Design review of the part built by this model. Coordinates are the model's own, in mm. Face numbers are marked on the shaded views. Give positions to 0.01 mm unless a question says otherwise; leave off trailing zeros. Write each loop counter-clockwise with the first axis right and the second up, starting at its lowest first coordinate (ties: lowest second). Pieces come first, ordered by that corner, then holes.
```python
from build123d import *

# Parameters (mm, degrees)
BASPROSKE_W         = 10
BASPROSKE_H         = 6
TOOTHCUT_DEPTH      = 14.114877049
TEETHCUTS_COUNT     = 10
TEETHCUTS_ANGLE     = 324
BORSKE_R            = 2.5
BORE_DEPTH          = 50.0000508
SKETCH1_R           = 2.5
BOSS_EXTRUDE1_DEPTH = 10
CUT_EXTRUDE2_DEPTH  = 10
CUT_EXTRUDE4_DEPTH  = 12.8
CUT_EXTRUDE5_DEPTH  = 7


with BuildPart() as part:
    # BasProSke → Base-Revolve (revolve)
    with BuildSketch(Plane(origin=(0, 0, 0), x_dir=(1, 0, 0), z_dir=(0, 1, 0)), mode=Mode.PRIVATE) as base_revolve_sk:
        with Locations((5, 3)):
            Rectangle(BASPROSKE_W, BASPROSKE_H)
    revolve(base_revolve_sk.sketch.rotate(Axis((-10, 0, 0), (1, 0, 0)), 180), axis=Axis((-10, 0, 0), (1, 0, 0)))

    # TooCutSke → ToothCut (cut, through all)
    with BuildSketch(Plane(origin=(0, 0, 0), x_dir=(0, 0, -1), z_dir=(1, 0, 0))):
        with BuildLine():
            ThreePointArc((0.59278292, 3.701838653), (0, 3.749), (-0.59278292, 3.701838653))
            ThreePointArc((-0.59278292, 3.701838653), (-0.846593509, 4.924114224), (-1.775771316, 5.757784417))
            ThreePointArc((-1.775771316, 5.757784417), (0, 6.0254), (1.775771316, 5.757784417))
            ThreePointArc((1.775771316, 5.757784417), (0.846593509, 4.924114224), (0.59278292, 3.701838653))
        make_face()
    toothcut = extrude(amount=TOOTHCUT_DEPTH, mode=Mode.SUBTRACT)

    # TeethCuts: ToothCut ×10 about axis
    teethcuts_axis = Axis((-10, 0, 0), (1, 0, 0))
    for i in range(1, TEETHCUTS_COUNT):
        add(toothcut.rotate(teethcuts_axis, i * TEETHCUTS_ANGLE / (TEETHCUTS_COUNT - 1)), mode=Mode.SUBTRACT)

    # BorSke → Bore (cut, symmetric)
    with BuildSketch(Plane(origin=(0, 0, 0), x_dir=(0, 0, -1), z_dir=(1, 0, 0))):
        with Locations(Location((0, 0, 0), (0, 0, 180))):
            Circle(BORSKE_R)
    extrude(amount=BORE_DEPTH, both=True, mode=Mode.SUBTRACT)

    # Sketch1 → Boss-Extrude1 (add)
    with BuildSketch(Plane(origin=(10, 0, 0), x_dir=(0, 0, -1), z_dir=(1, 0, 0))):
        Circle(SKETCH1_R)
    extrude(amount=-BOSS_EXTRUDE1_DEPTH)

    # Sketch2 → Cut-Extrude2 (cut)
    with BuildSketch(Plane.ZY):
        with BuildLine():
            Line((1.187434209, 2.2), (-1.187434209, 2.2))
            ThreePointArc((-1.187434209, 2.2), (-1.280900948, -2.146926352), (2.5, 0))
            ThreePointArc((2.5, 0), (2.146926352, 1.280900948), (1.187434209, 2.2))
        make_face()
    extrude(amount=-CUT_EXTRUDE2_DEPTH, mode=Mode.SUBTRACT)

    # Sketch3 → Cut-Extrude4 (cut)
    with BuildSketch(Plane.ZY):
        with BuildLine():
            ThreePointArc((-1.385640646, 2.2), (0, -2.6), (1.385640646, 2.2))
            Line((1.385640646, 2.2), (-1.385640646, 2.2))
        make_face()
    extrude(amount=-CUT_EXTRUDE4_DEPTH, mode=Mode.SUBTRACT)

    # Sketch4 → Cut-Extrude5 (cut)
    with BuildSketch(Plane(origin=(10, 0, 0), x_dir=(0, 0, -1), z_dir=(1, 0, 0))):
        with BuildLine():
            ThreePointArc((5.99882193, 0.11889261), (4.925863873, 0.720361677), (3.703837769, 0.580160996))
            ThreePointArc((3.703837769, 0.580160996), (3.56551088, 1.158504712), (3.337477777, 1.707701113))
            ThreePointArc((3.337477777, 1.707701113), (4.408525556, 2.3125653), (4.92303221, 3.429832919))
            ThreePointArc((4.92303221, 3.429832919), (4.854101966, 3.526711514), (4.783265565, 3.622205204))
            ThreePointArc((4.783265565, 3.622205204), (3.561689615, 3.478134978), (2.655457622, 2.646421322))
            ThreePointArc((2.655457622, 2.646421322), (2.203606911, 3.033004712), (1.69631471, 3.343279438))
            ThreePointArc((1.69631471, 3.343279438), (2.207280316, 4.462170935), (1.966811514, 5.668478849))
            ThreePointArc((1.966811514, 5.668478849), (1.854101966, 5.706339098), (1.740664331, 5.741958524))
            ThreePointArc((1.740664331, 5.741958524), (0.837070982, 4.907378935), (0.59278292, 3.701838653))
            ThreePointArc((0.59278292, 3.701838653), (0, 3.749), (-0.59278292, 3.701838653))
            ThreePointArc((-0.59278292, 3.701838653), (-0.837070982, 4.907378935), (-1.740664331, 5.741958524))
            ThreePointArc((-1.740664331, 5.741958524), (-1.854101966, 5.706339098), (-1.966811514, 5.668478849))
            ThreePointArc((-1.966811514, 5.668478849), (-2.207280316, 4.462170935), (-1.69631471, 3.343279438))
            ThreePointArc((-1.69631471, 3.343279438), (-2.203606911, 3.033004712), (-2.655457622, 2.646421322))
            ThreePointArc((-2.655457622, 2.646421322), (-3.561689615, 3.478134978), (-4.783265565, 3.622205204))
            ThreePointArc((-4.783265565, 3.622205204), (-4.854101966, 3.526711514), (-4.92303221, 3.429832919))
            ThreePointArc((-4.92303221, 3.429832919), (-4.408525556, 2.3125653), (-3.337477777, 1.707701113))
            ThreePointArc((-3.337477777, 1.707701113), (-3.56551088, 1.158504712), (-3.703837769, 0.580160996))
            ThreePointArc((-3.703837769, 0.580160996), (-4.925863873, 0.720361677), (-5.99882193, 0.11889261))
            ThreePointArc((-5.99882193, 0.11889261), (-6, 0), (-5.99882193, -0.11889261))
            ThreePointArc((-5.99882193, -0.11889261), (-4.925863873, -0.720361677), (-3.703837769, -0.580160996))
            ThreePointArc((-3.703837769, -0.580160996), (-3.56551088, -1.158504712), (-3.337477777, -1.707701113))
            ThreePointArc((-3.337477777, -1.707701113), (-4.408525556, -2.3125653), (-4.92303221, -3.429832919))
            ThreePointArc((-4.92303221, -3.429832919), (-4.854101966, -3.526711514), (-4.783265565, -3.622205204))
            ThreePointArc((-4.783265565, -3.622205204), (-3.561689615, -3.478134978), (-2.655457622, -2.646421322))
            ThreePointArc((-2.655457622, -2.646421322), (-2.203606911, -3.033004712), (-1.69631471, -3.343279438))
            ThreePointArc((-1.69631471, -3.343279438), (-2.207280316, -4.462170935), (-1.966811514, -5.668478849))
            ThreePointArc((-1.966811514, -5.668478849), (-1.854101966, -5.706339098), (-1.740664331, -5.741958524))
            ThreePointArc((-1.740664331, -5.741958524), (-0.837070982, -4.907378935), (-0.59278292, -3.701838653))
            ThreePointArc((-0.59278292, -3.701838653), (0, -3.749), (0.59278292, -3.701838653))
            ThreePointArc((0.59278292, -3.701838653), (0.837070982, -4.907378935), (1.740664331, -5.741958524))
            ThreePointArc((1.740664331, -5.741958524), (1.854101966, -5.706339098), (1.966811514, -5.668478849))
            ThreePointArc((1.966811514, -5.668478849), (2.207280316, -4.462170935), (1.69631471, -3.343279438))
            ThreePointArc((1.69631471, -3.343279438), (2.203606911, -3.033004712), (2.655457622, -2.646421322))
            ThreePointArc((2.655457622, -2.646421322), (3.561689615, -3.478134978), (4.783265565, -3.622205204))
            ThreePointArc((4.783265565, -3.622205204), (4.854101966, -3.526711514), (4.92303221, -3.429832919))
            ThreePointArc((4.92303221, -3.429832919), (4.408525556, -2.3125653), (3.337477777, -1.707701113))
            ThreePointArc((3.337477777, -1.707701113), (3.56551088, -1.158504712), (3.703837769, -0.580160996))
            ThreePointArc((3.703837769, -0.580160996), (4.925863873, -0.720361677), (5.99882193, -0.11889261))
            ThreePointArc((5.99882193, -0.11889261), (6, 0), (5.99882193, 0.11889261))
        make_face()
    extrude(amount=-CUT_EXTRUDE5_DEPTH, mode=Mode.SUBTRACT)


solid = part.part
```
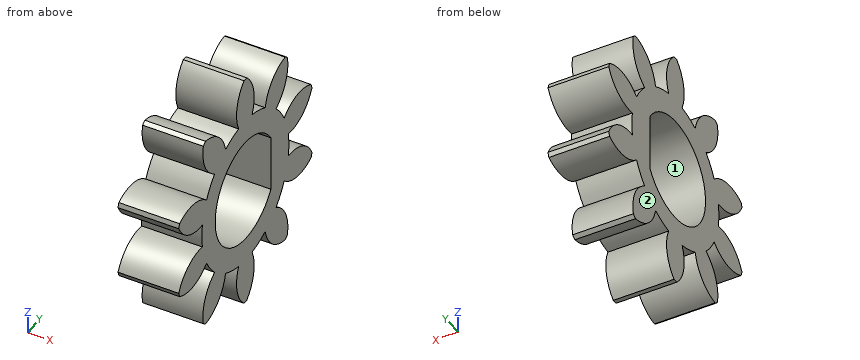
(1) Consider section B-B, the plane y = 1. Give the boundary of the cut face in (x, z), then the cut area to 3 significant figures.
Resolved:
outline: (0, -3.61) - (3, -3.61) - (3, -2.4) - (0, -2.4) - close; (0, 2.4) - (3, 2.4) - (3, 3.61) - (0, 3.61) - close
area: 7.28 mm2
(2) To check wall thickness, follow L1, parallel to Z at x = 0.75, y = 0; L2, parallel to Z at x = 2.7, y = -3.25; L3, parallel to Z at x = 2.85, y = 3. State the ranges of each line that lie inside material, in increasing order.
Resolved:
L1: z = -6 to -2.6, 2.6 to 6
L2: z = -4.89 to -3.18, -1.87 to 1.87, 3.18 to 4.89
L3: z = -4.82 to -2.91, -2.25 to 2.25, 2.91 to 4.82
(3) Consider section A-A, the plane z = 0. Give the boundary of the cut face in (x, y).
Resolved:
outline: (0, -3.75) - (3, -3.75) - (3, -2.6) - (0, -2.6) - close; (0, 2.2) - (3, 2.2) - (3, 3.75) - (0, 3.75) - close
(4) Clearance check with flat-ended pins moving along their axes: P1, Ø1.5, axis at x = 2.5, y = -0.5, coming from the +Z side; P2, Ø1.5, axis at x = 2, y = 2, coming from the +Z side. State where each tip first meets the part, or that it passes through.
Resolved:
P1: stops at z = 6
P2: stops at z = 4.71
(5) Mouldability with a two-part tool opening along Z and no side actions: class the marked faces 1 and 2 as pulls with the +Z half, pulls with the -Z half, needs draft (parallel to the pull), parting line crosses it, or undercut.
Resolved:
face 1: undercut
face 2: needs draft
(6) Consider section C-C, the plane z = 4. Give the boundary of the cut face in (x, y), then the cut area to 3 significant figures.
Resolved:
outline: (0, -3.62) - (3, -3.62) - (3, -1.97) - (0, -1.97) - close; (0, -0.69) - (3, -0.69) - (3, 0.69) - (0, 0.69) - close; (0, 1.97) - (3, 1.97) - (3, 3.62) - (0, 3.62) - close
area: 14.0 mm2
